from build123d import *

# Parameters (mm, degrees)
F0_W      = 215.9
F0_H      = 73.66
F0_W_2    = 205.74
F0_H_2    = 63.5
F1_DEPTH  = 5.08
F2_DEPTH  = 40.64
F3_R      = 1.64465
F4_DEPTH  = 5.081
F5_R      = 1.905
F6_DEPTH  = 12.7
F7_W      = 17.78
F7_H      = 21.336
F8_DEPTH  = 19.05
F9_W      = 17.78
F9_H      = 15.24
F9_H_2    = 21.336
F9_H_3    = 51.816
F10_DEPTH = 2.54
F11_R     = 3.175
F12_DEPTH = 2.54


with BuildPart() as f1:
    # F0 (on Top) → F1 (new body)
    with BuildSketch(Plane.XY):
        with Locations((55.0861711621, 20.7609453964)):
            Rectangle(F0_W, F0_H)
        with Locations((55.0861711621, 20.7609453964)):
            Rectangle(F0_W_2, F0_H_2, mode=Mode.SUBTRACT)
        with Locations((55.0861711621, 20.7609453964)):
            Rectangle(F0_W_2, F0_H_2)
    extrude(amount=-F1_DEPTH)

    # F0 (on Top) → F2 (join)
    with BuildSketch(Plane.XY):
        with Locations((55.0861711621, 20.7609453964)):
            Rectangle(F0_W, F0_H)
        with Locations((55.0861711621, 20.7609453964)):
            Rectangle(F0_W_2, F0_H_2, mode=Mode.SUBTRACT)
    extrude(amount=F2_DEPTH)

    # F3 (on face) → F4 (cut, through all)
    with BuildSketch(Plane.XY):
        with Locations((150.1329711621, 29.7802567964)):
            Circle(F3_R)
        with Locations((150.1329711621, 2.8943567964)):
            Circle(F3_R)
        with Locations((100.6029711621, -2.4650432036)):
            Circle(F3_R)
        with Locations((99.6123711621, 44.7766453964)):
            Circle(F3_R)
    extrude(amount=-F4_DEPTH, mode=Mode.SUBTRACT)

    # F5 (on face) → F6 (cut)
    with BuildSketch(Plane.XY.offset(40.64)):
        with Locations((160.4961711621, -13.5290546036)):
            Circle(F5_R)
        with Locations((160.4961711621, 55.0509453964)):
            Circle(F5_R)
        with Locations((-50.3238288379, 55.0509453964)):
            Circle(F5_R)
        with Locations((-50.3238288379, -13.5290546036)):
            Circle(F5_R)
    extrude(amount=-F6_DEPTH, mode=Mode.SUBTRACT)

    # F7 (on face) → F8 (join)
    with BuildSketch(Plane(origin=(0, 0, -5.08), x_dir=(1, 0, 0), z_dir=(0, 0, -1))):
        with Locations((128.7461711621, -20.7609453964)):
            Rectangle(F7_W, F7_H)
        with Locations((-18.5738288379, -20.7609453964)):
            Rectangle(F7_W, F7_H)
    extrude(amount=F8_DEPTH)

    # F9 (on face) → F10 (join)
    with BuildSketch(Plane(origin=(0, 0, -24.13), x_dir=(1, 0, 0), z_dir=(0, 0, -1))):
        with Locations((128.7461711621, -39.0489453964)):
            Rectangle(F9_W, F9_H)
        with Locations((128.7461711621, -20.7609453964)):
            Rectangle(F9_W, F9_H_2)
        with Locations((128.7461711621, -2.4729453964)):
            Rectangle(F9_W, F9_H)
        with Locations((-18.5738288379, -20.7609453964)):
            Rectangle(F9_W, F9_H_3)
    extrude(amount=F10_DEPTH)

    # F11 (on face) → F12 (cut, through all)
    with BuildSketch(Plane(origin=(0, 0, -26.67), x_dir=(1, 0, 0), z_dir=(0, 0, -1))):
        with Locations((-18.5738288379, -1.2029453964)):
            Circle(F11_R)
        with Locations((-18.5738288379, -40.3189453964)):
            Circle(F11_R)
        with Locations((128.7461711621, -40.3189453964)):
            Circle(F11_R)
        with Locations((128.7461711621, -1.2029453964)):
            Circle(F11_R)
    extrude(amount=-F12_DEPTH, mode=Mode.SUBTRACT)


solid = f1.part
The listing builds one solid part. Answer for the finished solid, in the listing's coordinates (mm). A direction names the side the tool comes from. Give positions to 0.01 mm unless a question says otherwise; leave off trailing zeros. Loops run counter-clockwise (first coordinate to the right, second up) from the corner with the lowest first, then second, coordinate; pieces in that order, holes last. Notation, with made-up numbers: (83, -26) - (115, -26) arc R10 ccw to (115, -11) - close; hole circle Ø1 at (-2.75, 55.25). An arc over 180 degrees is marked (long way). Use one line per item in the form item = value.
1. Section B-B on y = 33.5 is taken. Give the vertices of the cut face in (x, z).
Calculated:
outline = (-52.86, -5.08) - (163.04, -5.08) - (163.04, 40.64) - (157.96, 40.64) - (157.96, 0) - (-47.78, 0) - (-47.78, 40.64) - (-52.86, 40.64) - close; (-27.46, -26.67) - (-9.68, -26.67) - (-9.68, -24.13) - (-27.46, -24.13) - close; (119.86, -26.67) - (137.64, -26.67) - (137.64, -24.13) - (119.86, -24.13) - close
2. The mould has two halves that part along Z. Classify faces 1 (the face through (129, 31.429, -14)), 2 (the face through (129, 20, -26.67)), 3 (the face through (162.313, 55.623, 34.379)), 4 (the face through (160, -14, 27.94)): pulls with the +Z half, pulls with the -Z half, needs draft (parallel to the pull), parting line crosses it, or undercut.
Calculated:
face_1 = undercut
face_2 = pulls with the -Z half
face_3 = needs draft
face_4 = pulls with the +Z half
3. Section D-D on x = 68.5 is taken. Give the vertices of the cut face in (y, z).
Calculated:
outline = (-16.07, -5.08) - (57.59, -5.08) - (57.59, 40.64) - (52.51, 40.64) - (52.51, 0) - (-10.99, 0) - (-10.99, 40.64) - (-16.07, 40.64) - close
4. Section A-A on z = -19 is taken. Give the vertices of the cut face in (x, y).
Calculated:
outline = (-27.46, 10.09) - (-9.68, 10.09) - (-9.68, 31.43) - (-27.46, 31.43) - close; (119.86, 10.09) - (137.64, 10.09) - (137.64, 31.43) - (119.86, 31.43) - close
5. Which of the six approach directions +Z, -Z, +X, -X, +Y, -Y give full straight-line access (tool end or side, diameter ignored) to faces 5 (the face through (-19, 31.429, -14)), 6 (the face through (-9.684, 21, -18)), 7 (the face through (54, 52.511, 20)), 8 (the face through (129, 10.093, -14))?
Calculated:
face_5 = +X, -X, +Y
face_6 = -Z, +Y, -Y
face_7 = +Z
face_8 = +X, -X, -Y
6. Given pin 1 Ø2 at (x, z) = (126, -25) entering from -Y; pin 2 Ø17 at (x, y) = (127, 2.5) entering from +Z; pin 3 Ø5 at (x, y) = (128.75, 40.32) entering from -Z; pin 4 Ø3 at (x, y) = (161.5, -12.5) entering from +Z, each flat-ended and moving along its own axis, determine where each tip first touches the part or whether it passes through.
Calculated:
pin_1 = -5.15
pin_2 = 0
pin_3 = -5.08
pin_4 = 40.64
7. Find the intervals of material crossed by line 1 along X through (y, z) = (-7, 37.5); line 2 along Y through (x, z) = (-37.5, 14); line 3 along Z through (x, y) = (138, 8.5), in increasing order. Write a range as [from, to].
Calculated:
line_1 = [-52.86, -47.78], [157.96, 163.04]
line_2 = [-16.07, -10.99], [52.51, 57.59]
line_3 = [-5.08, 0]
8. Section C-C on z = 25 is taken. Give the vertices of the cut face in (x, y).
Calculated:
outline = (-52.86, -16.07) - (163.04, -16.07) - (163.04, 57.59) - (-52.86, 57.59) - close; hole (-47.78, -10.99) - (157.96, -10.99) - (157.96, 52.51) - (-47.78, 52.51) - close
